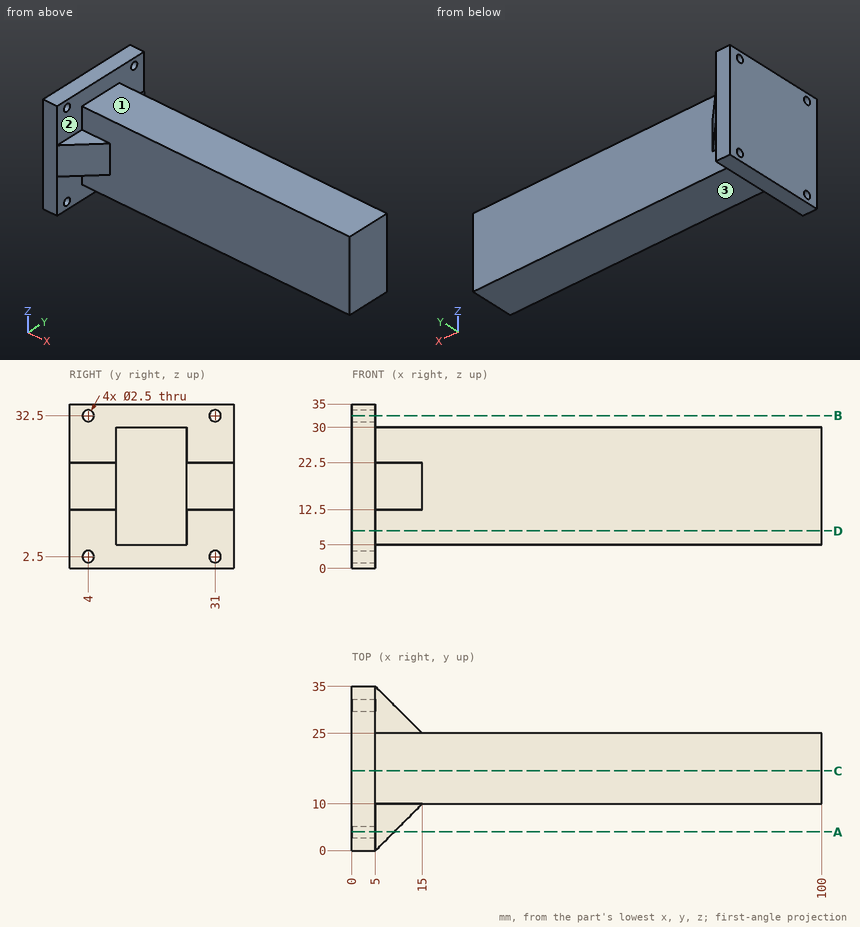
Answer from the drawing. Dimensions are ordinates in mm from the lowest x, y and z of the part. Give positions to 0.01 mm unless a question says otherwise; leave off trailing zeros. Order: outer loops, then holes, each group sorted by start corner. A loop starts at its lowest first (then second) coordinate and runs counter-clockwise, first axis right, second up. Notation, with made-up numbers: (5.25, 7.5) - (44.25, 7.5) arc R15 cw to (44.25, 18.5) - close; hole circle Ø9 at (-11.5, 17.5). An arc over 180 degrees is marked (long way). One line per item, written item: value. Start each with the question number.
1. For a pull along Z with two mould halves and no side action, classify the marked faces 1, 2 and 3 as released by +Z, released by -Z, zero draft, split by the parting line, or undercut.
2. Each of these flat-tipped pins is pushed along its axis until it touches: pin 1 Ø11 at (x, y) = (12, 29) entering from -Z; pin 2 Ø12.5 at (x, z) = (41.5, 18.5) entering from -Y; pin 3 Ø7.5 at (x, y) = (60, 18) entering from +Z. Where does it stop, or does it pass through?
3. Section B-B, the plane z = 32.5 is taken. Write down the section's boundary in (x, y).
4. Consider line 1 (Y direction, x = 2.95, z = 2.5); line 2 (Y direction, x = 94.5, z = 20); line 3 (X direction, y = 7.5, z = 27). Determine where each line is inside the solid, lowest interval first.
5. Section A-A, the plane y = 4 is taken. Write down the section's boundary in (x, z), then the cut area to 3 significant figures.
6. Section C-C, the plane y = 17 is taken. Write down the section's boundary in (x, z), then the cut area to 3 significant figures.
7. Section D-D, the plane z = 8 is taken. Write down the section's boundary in (x, y), then the cut area to 3 significant figures.
Filled sheet:
1. face 1: released by +Z
1. face 2: zero draft
1. face 3: released by -Z
2. pin 1: z = 5
2. pin 2: y = 10
2. pin 3: z = 30
3. outline: (0, 0) - (5, 0) - (5, 2.75) - (0, 2.75) - close; (0, 5.25) - (5, 5.25) - (5, 29.75) - (0, 29.75) - close; (0, 32.25) - (5, 32.25) - (5, 35) - (0, 35) - close
4. line 1: 0 to 2.75, 5.25 to 29.75, 32.25 to 35
4. line 2: 10 to 25
4. line 3: 0 to 5
5. outline: (0, 0) - (5, 0) - (5, 1.25) - (0, 1.25) - close; (0, 3.75) - (5, 3.75) - (5, 12.5) - (9, 12.5) - (9, 22.5) - (5, 22.5) - (5, 31.25) - (0, 31.25) - close; (0, 33.75) - (5, 33.75) - (5, 35) - (0, 35) - close
5. area: 190 mm²
6. outline: (0, 0) - (5, 0) - (5, 5) - (100, 5) - (100, 30) - (5, 30) - (5, 35) - (0, 35) - close
6. area: 2,550 mm²
7. outline: (0, 0) - (5, 0) - (5, 10) - (100, 10) - (100, 25) - (5, 25) - (5, 35) - (0, 35) - close
7. area: 1,600 mm²
